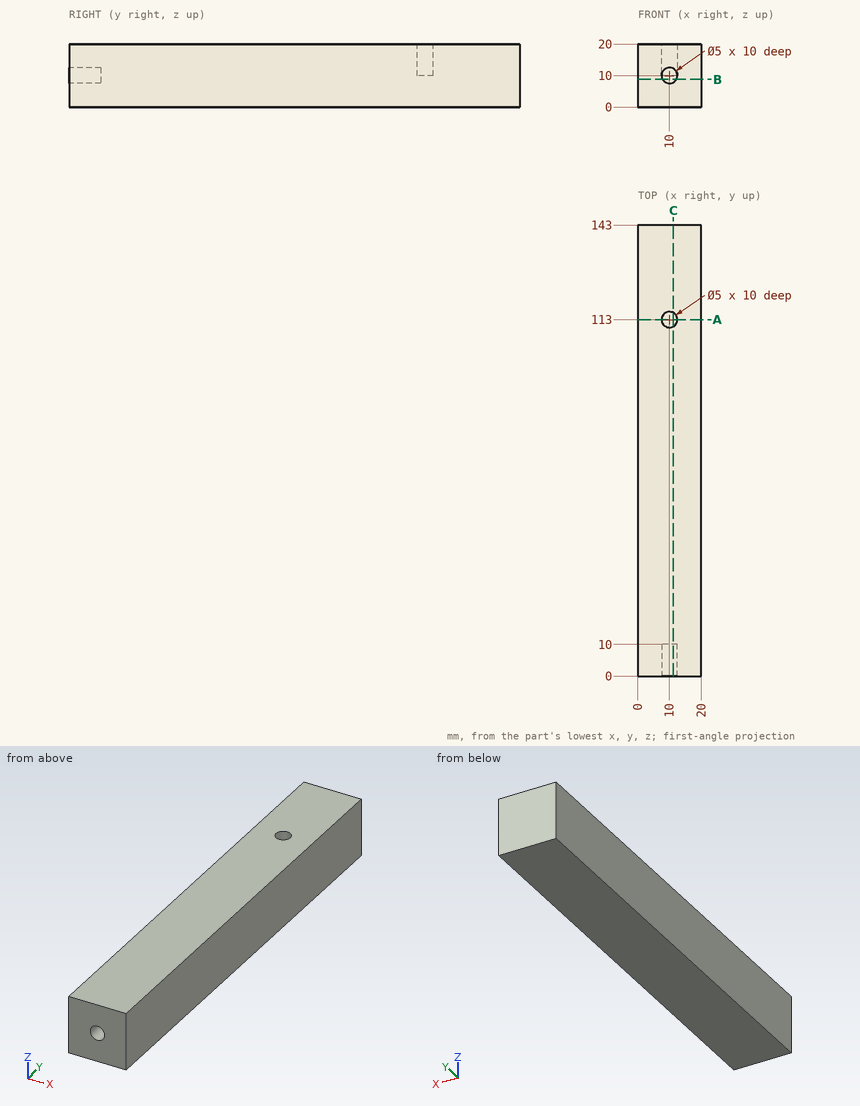
Input: dimensioned drawing with shaded views. Units: mm. Origin: part minimum x, y, z. Give positions to 0.01 mm unless a question says otherwise; leave off trailing zeros. Write each loop counter-clockwise with the first axis right and the second up, starting at its lowest first coordinate (ties: lowest second). Pieces come first, ordered by that corner, then holes.
1. Section query B-B, the plane z = 8.75. Return loops of the section in (x, y).
2. Section query C-C, the plane x = 11.25. Return loops of the section in (y, z).
3. Line query: probe 1 along Z at (x, y) = (10, 6.5); probe 2 along Y at (x, z) = (10, 18); probe 3 along Z at (x, y) = (10, 113). Output: solid intervals per line, ascending.
4. Section query A-A, the plane y = 113. Return loops of the section in (x, z), then the cut area to 3 significant figures.
Computed:
1. outline: (0, 0) - (7.83, 0) - (7.83, 10) - (12.17, 10) - (12.17, 0) - (20, 0) - (20, 143) - (0, 143) - close
2. outline: (0, 0) - (143, 0) - (143, 20) - (115.17, 20) - (115.17, 10) - (110.83, 10) - (110.83, 20) - (0, 20) - (0, 12.17) - (10, 12.17) - (10, 7.83) - (0, 7.83) - close
3. probe 1: z = 0 to 7.5, 12.5 to 20
3. probe 2: y = 0 to 110.5, 115.5 to 143
3. probe 3: z = 0 to 10
4. outline: (0, 0) - (20, 0) - (20, 20) - (12.5, 20) - (12.5, 10) - (7.5, 10) - (7.5, 20) - (0, 20) - close
4. area: 350 mm2
